Could you check a few things on this model? Use its own coordinates, in mm. A direction names the side the tool comes from. Round coordinates to 2 decimals unless told otherwise and drop trailing zeros. Loops run counter-clockwise (first coordinate to the right, second up) from the corner with the lowest first, then second, coordinate; pieces in that order, holes last.
from build123d import *

# Parameters (mm, degrees)
F1_DEPTH  = 45
F2_W      = 216.5675759315
F2_H      = 199.976965785
F2_W_2    = 183.3030277982
F2_H_2    = 45
F3_DEPTH  = 35
F4_W      = 45
F4_H      = 45
F5_DEPTH  = 20
F6_R      = 17.5
F7_DEPTH  = 25
F8_R      = 14.5
F9_DEPTH  = 18
F10_W     = 7
F10_H     = 9
F11_DEPTH = 10
F12_W     = 35
F12_H     = 20
F13_DEPTH = 140
F15_DEPTH = 113.8973534547
F16_SIZE  = 5
F17_SIZE  = 3
F18_W     = 20
F18_H     = 4
F19_DEPTH = 10
F21_DEPTH = 113.8973534547


with BuildPart() as f1:
    # F0 (on Top) → F1 (new body)
    with BuildSketch(Plane.XY):
        Polygon((-91.6515138991, 22.5), (-91.6515138991, -22.5), (-59.9372190952, -22.5), (-23.3139814323, -22.5), (23.3139814323, -22.5), (59.9372190952, -22.5), (91.6515138991, -22.5), (91.6515138991, 22.5), (59.9372190952, 22.5), (23.3139814323, 22.5), (-23.3139814323, 22.5), (-59.9372190952, 22.5), align=None)
        with BuildLine():
            Line((-23.3139814323, -22.5), (-59.9372190952, -22.5))
            Line((-59.9372190952, -22.5), (-91.6515138991, -67.7927069095))
            ThreePointArc((-91.6515138991, -67.7927069095), (-74.8536462422, -62.0905991935), (-64.3642332348, -76.3963534547))
            ThreePointArc((-64.3642332348, -76.3963534547), (-65.0584789736, -80.9069404473), (-67.0769525704, -85))
            Line((-67.0769525704, -85), (-23.3139814323, -22.5))
        make_face()
        with BuildLine():
            ThreePointArc((-64.3642332348, -76.3963534547), (-74.8536462422, -62.0905991935), (-91.6515138991, -67.7927069095))
            Line((-91.6515138991, -67.7927069095), (-67.0769525704, -85))
            ThreePointArc((-67.0769525704, -85), (-65.0584789736, -80.9069404473), (-64.3642332348, -76.3963534547))
        make_face()
        with BuildLine():
            Line((-67.0769525704, -85), (-91.6515138991, -67.7927069095))
            ThreePointArc((-91.6515138991, -67.7927069095), (-87.96787978, -88.6836341191), (-67.0769525704, -85))
        make_face()
        with BuildLine():
            Line((-91.6515138991, 67.7927069095), (-59.9372190952, 22.5))
            Line((-59.9372190952, 22.5), (-23.3139814323, 22.5))
            Line((-23.3139814323, 22.5), (-67.0769525704, 85))
            ThreePointArc((-67.0769525704, 85), (-65.0584789736, 80.9069404473), (-64.3642332348, 76.3963534547))
            ThreePointArc((-64.3642332348, 76.3963534547), (-74.8536462422, 62.0905991935), (-91.6515138991, 67.7927069095))
        make_face()
        with BuildLine():
            Line((59.9372190952, -22.5), (23.3139814323, -22.5))
            Line((23.3139814323, -22.5), (67.0769525704, -85))
            ThreePointArc((67.0769525704, -85), (70.7605866895, -64.1090727904), (91.6515138991, -67.7927069095))
            Line((91.6515138991, -67.7927069095), (59.9372190952, -22.5))
        make_face()
        with BuildLine():
            ThreePointArc((-67.0769525704, 85), (-87.96787978, 88.6836341191), (-91.6515138991, 67.7927069095))
            ThreePointArc((-91.6515138991, 67.7927069095), (-74.8536462422, 62.0905991935), (-64.3642332348, 76.3963534547))
            ThreePointArc((-64.3642332348, 76.3963534547), (-65.0584789736, 80.9069404473), (-67.0769525704, 85))
        make_face()
        with BuildLine():
            ThreePointArc((91.6515138991, -67.7927069095), (70.7605866895, -64.1090727904), (67.0769525704, -85))
            ThreePointArc((67.0769525704, -85), (83.8748202273, -90.702107716), (94.3642332348, -76.3963534547))
            ThreePointArc((94.3642332348, -76.3963534547), (93.669987496, -71.8857664622), (91.6515138991, -67.7927069095))
        make_face()
        with BuildLine():
            Line((67.0769525704, 85), (23.3139814323, 22.5))
            Line((23.3139814323, 22.5), (59.9372190952, 22.5))
            Line((59.9372190952, 22.5), (91.6515138991, 67.7927069095))
            ThreePointArc((91.6515138991, 67.7927069095), (70.7605866895, 64.1090727904), (67.0769525704, 85))
        make_face()
        with BuildLine():
            ThreePointArc((94.3642332348, 76.3963534547), (83.8748202273, 90.702107716), (67.0769525704, 85))
            ThreePointArc((67.0769525704, 85), (70.7605866895, 64.1090727904), (91.6515138991, 67.7927069095))
            ThreePointArc((91.6515138991, 67.7927069095), (93.669987496, 71.8857664622), (94.3642332348, 76.3963534547))
        make_face()
    extrude(amount=F1_DEPTH)

    # F2 (on face) → F3 (cut)
    with BuildSketch(Plane.XY.offset(45)):
        Rectangle(F2_W, F2_H)
        Rectangle(F2_W_2, F2_H_2, mode=Mode.SUBTRACT)
    extrude(amount=-F3_DEPTH, mode=Mode.SUBTRACT)

    # F4 (on face) → F5 (cut)
    with BuildSketch(Plane.YZ.offset(91.6515138991)):
        with Locations((0, 22.5)):
            Rectangle(F4_W, F4_H)
    extrude(amount=-F5_DEPTH, mode=Mode.SUBTRACT)

    # F6 (on face) → F7 (join)
    with BuildSketch(Plane.YZ.offset(71.6515138991)):
        with Locations((0, 10)):
            Circle(F6_R)
    extrude(amount=-F7_DEPTH)

    # F8 (on face) → F9 (cut)
    with BuildSketch(Plane.YZ.offset(71.6515138991)):
        with Locations((0, 10)):
            Circle(F8_R)
    extrude(amount=-F9_DEPTH, mode=Mode.SUBTRACT)

    # F10 (on face) → F11 (cut)
    with BuildSketch(Plane.YZ.offset(53.6515138991)):
        with Locations((0, 24.5)):
            Rectangle(F10_W, F10_H)
    extrude(amount=-F11_DEPTH, mode=Mode.SUBTRACT)

    # F12 (on face) → F13 (cut)
    with BuildSketch(Plane(origin=(-91.6515138991, 0, 0), x_dir=(0, -1, 0), z_dir=(-1, 0, 0))):
        with Locations((0, 20)):
            Rectangle(F12_W, F12_H)
    extrude(amount=-F13_DEPTH, mode=Mode.SUBTRACT)

    # F14 (on face) → F15 (cut, through all)
    with BuildSketch(Plane(origin=(0, 22.5, 0), x_dir=(-1, 0, 0), z_dir=(0, 1, 0))):
        Polygon((-21.6515138991, 69.95960325), (-21.6515138991, 45), (-6.6515138991, 35), (91.6515138991, 35), (106.8655148461, 35), (106.8655148461, 69.95960325), align=None)
    extrude(amount=-F15_DEPTH, mode=Mode.SUBTRACT)

    # F16
    f16_edges = [f1.edges().sort_by_distance(p)[0] for p in [
        (46.651514, 22.5, 45),
        (46.651514, -22.5, 45),
        (14.151514, -22.5, 40),
        (14.151514, 22.5, 40),
        (-42.5, 22.5, 35),
        (-42.5, -22.5, 35),
    ]]
    chamfer(f16_edges, length=F16_SIZE)

    # F17
    f17_edges = [f1.edges().sort_by_distance(p)[0] for p in [
        (-21.651514, 17.5, 30),
        (-21.651514, -17.5, 30),
    ]]
    chamfer(f17_edges, length=F17_SIZE)

    # F18 (on face) → F19 (cut)
    with BuildSketch(Plane.XY.offset(35)):
        with Locations((-78.6515138991, 12.5)):
            Rectangle(F18_W, F18_H)
        with Locations((-43.6515138991, 12.5)):
            Rectangle(F18_W, F18_H)
        with Locations((-8.6515138991, 12.5)):
            Rectangle(F18_W, F18_H)
        with Locations((-78.6515138991, -12.5)):
            Rectangle(F18_W, F18_H)
        with Locations((-8.6515138991, -12.5)):
            Rectangle(F18_W, F18_H)
        with Locations((-43.6515138991, -12.5)):
            Rectangle(F18_W, F18_H)
    extrude(amount=-F19_DEPTH, mode=Mode.SUBTRACT)

    # F20 (on face) → F21 (cut, through all)
    with BuildSketch(Plane.XZ.offset(22.5)):
        Polygon((-51.6515138991, 30), (-76.6515138991, 30), (-87.6515138991, 15.3333333333), (-87.6515138991, 10), (-66.6515138991, 10), align=None)
        Polygon((-1.6515138991, 30), (-26.6515138991, 30), (-41.6515138991, 10), (-23.3139814323, 10), (-16.6515138991, 10), align=None)
        Polygon((48.3484861009, 30), (23.3484861009, 30), (8.3484861009, 10), (23.3139814323, 10), (33.3484861009, 10), align=None)
    extrude(amount=-F21_DEPTH, mode=Mode.SUBTRACT)


solid = f1.part
Item 1: If we section it at D-D, the plane y = 80.5: Please give me the cut outline in (x, z), then the cut area to 3 significant figures.
Results list:
outline: (-93.79, 0) - (-63.93, 0) - (-63.93, 10) - (-93.79, 10) - close; (63.93, 0) - (93.79, 0) - (93.79, 10) - (63.93, 10) - close
area: 597 mm2
Item 2: If we section it at B-B, the plane x = 82.5: Please give me the cut outline in (y, z).
Results list:
outline: (-91.06, 0) - (-54.72, 0) - (-54.72, 10) - (-91.06, 10) - close; (54.72, 0) - (91.06, 0) - (91.06, 10) - (54.72, 10) - close
Item 3: Will these pins go through, and if not, where does the flat tip stop? pin 1 (4.5 mm diameter, centred on y = -13.5, z = 33, fed in from +X); pin 2 (1.5 mm diameter, centred on x = -75.5, z = 33.5, fed in from -Y); pin 3 (12 mm diameter, centred on x = 44, z = 22, fed in from -Y).
Results list:
pin 1: stops at x = 71.65
pin 2: stops at y = -19.75
pin 3: stops at y = -22.5
Item 4: If I drill on line 1 along Z through (x, y) = (34, -8); line 2 along Z through (x, y) = (66.5, 0); line 3 along Y through (x, z) = (-62, 15), over which ranges is the centre line in solid material (lowest first)?
Results list:
line 1: z = 0 to 10, 30 to 45
line 2: z = -7.5 to -4.5, 24.5 to 45
line 3: y = -22.5 to -17.5, 17.5 to 22.5
Item 5: If we section it at A-A, the plane y = 0: Please give me the cut outline in (x, z), then the cut area to 3 significant figures.
Results list:
outline: (-91.65, 0) - (46.65, 0) - (46.65, -7.5) - (71.65, -7.5) - (71.65, -4.5) - (53.65, -4.5) - (53.65, 20) - (48.35, 20) - (48.35, 10) - (-91.65, 10) - close; (-91.65, 30) - (48.35, 30) - (48.35, 29) - (53.65, 29) - (53.65, 24.5) - (71.65, 24.5) - (71.65, 45) - (21.65, 45) - (6.65, 35) - (-91.65, 35) - close
area: 3,110 mm2
Item 6: For faces 1 (the flat face through (-23, 0, 30)), 2 (the flat face through (-34.047, -19.445, 20.14)), 3 (the flat face through (-42, 0, 35)), which set-ups out of +Z, -Z, +X, -X, +Y, -Y let a thin tool reach every point of the face, with its end or its side?
Results list:
face 1: none
face 2: +Y, -Y
face 3: +Z, -X, +Y, -Y
Item 7: If we section it at C-C, the plane x = 57: Please give me the cut outline in (y, z).
Results list:
outline: (-70.61, 0) - (-14.36, 0) arc R17.5 ccw to (14.36, 0) - (70.61, 0) - (70.61, 10) - (22.5, 10) - (22.5, 40) - (17.5, 45) - (-17.5, 45) - (-22.5, 40) - (-22.5, 10) - (-70.61, 10) - close; hole circle Ø29 at (0, 10)
Item 8: We'd pull the mould along X, two halves only. Please class faces 4 (the flat face through (-9.257, -19.445, 19.86)), 5 (the flat face through (14.3, 0.2, 40.1)), 6 (the flat face through (75.572, 44.829, 4.93)): released by +X, released by -X, zero draft, split by the parting line, or undercut.
Results list:
face 4: undercut
face 5: released by -X
face 6: released by +X
